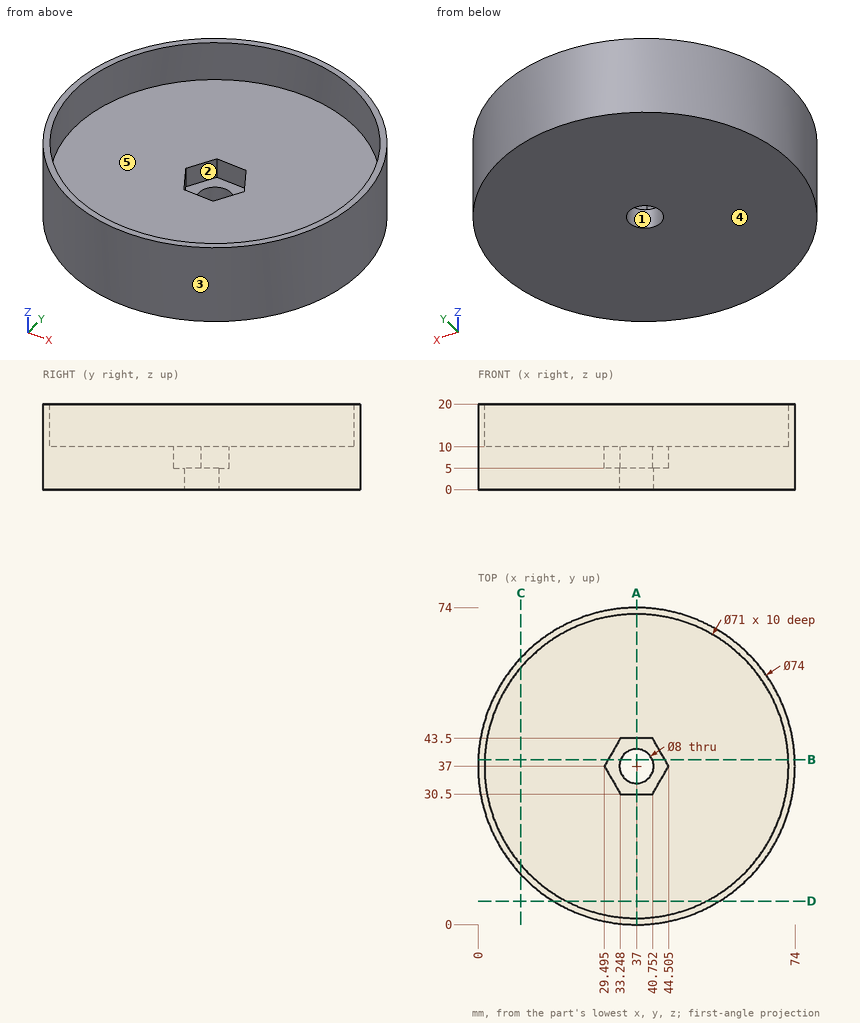
Print and shaded views of the part. All mm, measured from the part's lowest x, y and z. A direction names the side the tool comes from. Give positions to 0.01 mm unless a question says otherwise; leave off trailing zeros. Write each loop counter-clockwise with the first axis right and the second up, starting at its lowest first coordinate (ties: lowest second). Pieces come first, ordered by that corner, then holes. Notation, with made-up numbers: M 59,-13.5 L 64,-13.5 A30 ccw 64,17.5 Z; hole C -13,59.5 d6. An arc over 180 degrees is marked long. Use a Markdown table: item, result.
1) Cut at A-A (x = 37). List the corners of the cut face in (y, z).
Responses:
| item | result |
|---|---|
| outline | M 0,0 L 33,0 L 33,5 L 30.5,5 L 30.5,10 L 1.5,10 L 1.5,20 L 0,20 Z; M 41,0 L 74,0 L 74,20 L 72.5,20 L 72.5,10 L 43.5,10 L 43.5,5 L 41,5 Z |
2) Cut at D-D (y = 5.5). List the corners of the cut face in (x, z), and give its area (3 significant figures).
Responses:
| item | result |
|---|---|
| outline | M 17.59,0 L 56.41,0 L 56.41,20 L 53.37,20 L 53.37,10 L 20.63,10 L 20.63,20 L 17.59,20 Z |
| area | 449 mm2 |
3) Cut at B-B (y = 38.5). List the corners of the cut face in (x, z).
Responses:
| item | result |
|---|---|
| outline | M 0.03,0 L 33.29,0 L 33.29,5 L 30.36,5 L 30.36,10 L 1.53,10 L 1.53,20 L 0.03,20 Z; M 40.71,0 L 73.97,0 L 73.97,20 L 72.47,20 L 72.47,10 L 43.64,10 L 43.64,5 L 40.71,5 Z |
4) Tool access for the marked faces 1 and 2: list every direction of +Z, -Z, +X, -X, +Y, -Y with a clear straight run to the whole face (end or side of a thin tool).
Responses:
| item | result |
|---|---|
| face 1 | +Z, -Z |
| face 2 | +Z |
5) Cut at C-C (x = 10). List the corners of the cut face in (y, z), and give its area (3 significant figures).
Responses:
| item | result |
|---|---|
| outline | M 11.7,0 L 62.3,0 L 62.3,20 L 60.05,20 L 60.05,10 L 13.95,10 L 13.95,20 L 11.7,20 Z |
| area | 551 mm2 |
6) Drill centre lines: line 1 (Y direction, x = 37, z = 17.25); line 2 (Z direction, x = 51.5, y = 15); line 3 (Y direction, x = 20, z = 11.25) (1 decimal). Where is each one in solid material? Low to high. Write a range as from..to.
Responses:
| item | result |
|---|---|
| line 1 | y = 0..1.5, 72.5..74 |
| line 2 | z = 0..10 |
| line 3 | y = 4.1..5.8, 68.2..69.9 |
7) Pull direction X, two halves, no side cores. Call the marked faces 3, 4 and 5: +X half, -X half, draft (parallel to the pull), parting line (faces both ways), or undercut.
Responses:
| item | result |
|---|---|
| face 3 | parting line |
| face 4 | draft |
| face 5 | undercut |
8) Pin check, flat tips, straight feed: pin 1 (2 mm diameter, centred on y = 28.5, z = 8.5, fed in from +X); pin 2 (4 mm diameter, centred on x = 37.5, z = 7, fed in from +Y); pin 3 (1 mm diameter, centred on x = 38, y = 66, fed in from +Z); pin 4 (1.5 mm diameter, centred on x = 66.5, y = 56, fed in from -Z). Stop position of each tip, or through.
Responses:
| item | result |
|---|---|
| pin 1 | stops at x = 73.23 |
| pin 2 | stops at y = 74 |
| pin 3 | stops at z = 10 |
| pin 4 | stops at z = 0 |
